Answer from the drawing. Dimensions are ordinates in mm from the lowest x, y and z of the part. Give positions to 0.01 mm unless a question says otherwise; leave off trailing zeros. Order: outer loops, then holes, each group sorted by start corner. A loop starts at its lowest first (then second) coordinate and runs counter-clockwise, first axis right, second up. Notation, with made-up numbers: (77, -16.75) -> (119, -16.75) arc R20 ccw to (119, 9.25) -> close; hole circle Ø7 at (39.5, 28.5). An arc over 180 degrees is marked (long way). Write item = value, one per line. Start each with the question number.
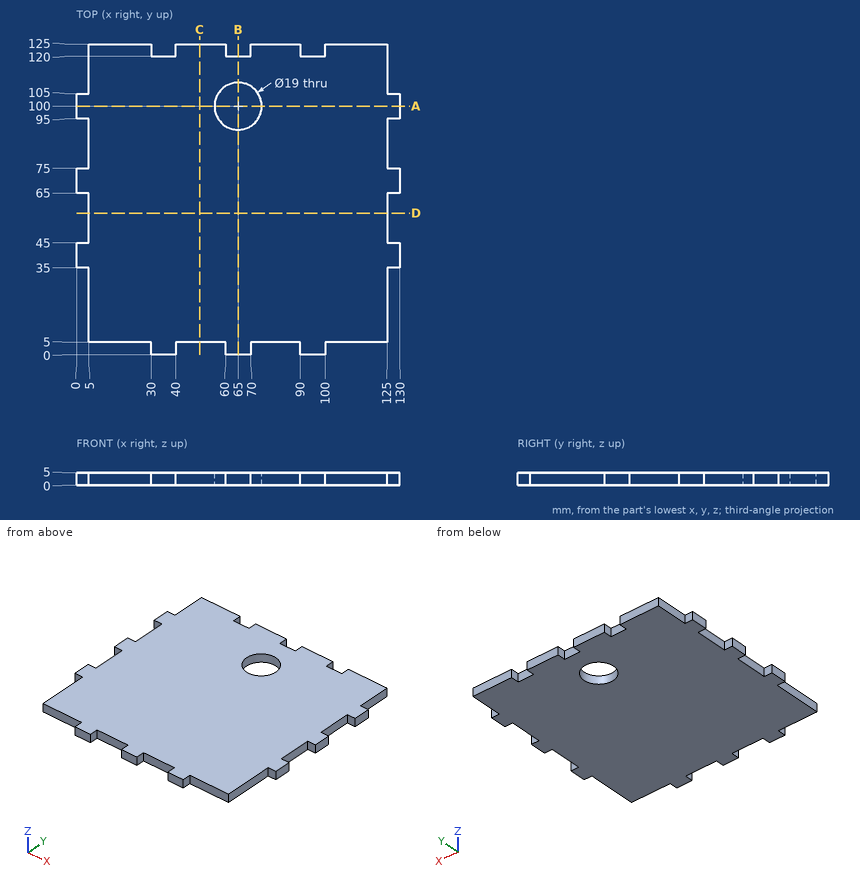
Item 1: Flat-ended cylindrical pins translate along their axes: pin 1 (1.5 mm diameter, centred on x = 126.5, z = 2.5, fed in from -Y); pin 2 (3 mm diameter, centred on y = 17, z = 3.5, fed in from +X); pin 3 (15 mm diameter, centred on x = 65, y = 100, fed in from -Z); pin 4 (3 mm diameter, centred on x = 16, z = 3, fed in from -Y). Find the tip coordinate at first contact, or state that the pin passes through.
Item 2: A cutting plane is placed at B-B, the plane x = 65. Write down the section's boundary in (y, z).
Item 3: A cutting plane is placed at C-C, the plane x = 49.5. Write down the section's boundary in (y, z), plus the area to 3 significant figures.
Item 4: A cutting plane is placed at A-A, the plane y = 100. Write down the section's boundary in (x, z).
Item 5: Consider L1, parallel to Y at x = 65, z = 2.55; L2, parallel to Y at x = 8, z = 4.5; L3, parallel to X at y = 103, z = 3.95. Determine where each line is inside the solid, lowest interval first. Write a range as from..to.
Check values:
q1.pin_1 = 35
q1.pin_2 = 125
q1.pin_3 = through
q1.pin_4 = 5
q2.outline = (0, 0) -> (90.5, 0) -> (90.5, 5) -> (0, 5) -> close; (109.5, 0) -> (120, 0) -> (120, 5) -> (109.5, 5) -> close
q3.outline = (5, 0) -> (125, 0) -> (125, 5) -> (5, 5) -> close
q3.area = 600 mm^2
q4.outline = (0, 0) -> (55.5, 0) -> (55.5, 5) -> (0, 5) -> close; (74.5, 0) -> (130, 0) -> (130, 5) -> (74.5, 5) -> close
q5.L1 = 0..90.5, 109.5..120
q5.L2 = 5..125
q5.L3 = 0..55.99, 74.01..130
